from build123d import *

# Parameters (mm, degrees)
SKETCH1_W           = 23
SKETCH1_H           = 31
BOSS_EXTRUDE1_DEPTH = 4
SKETCH2_W           = 10
SKETCH2_H           = 31
BOSS_EXTRUDE2_DEPTH = 2
SKETCH3_R           = 1
CUT_EXTRUDE1_DEPTH  = 24
FILLET1_R           = 2
FILLET2_R           = 6
FILLET3_R           = 0.762


with BuildPart() as part:
    # Sketch1 → Boss-Extrude1 (new body)
    with BuildSketch(Plane.XY):
        Rectangle(SKETCH1_W, SKETCH1_H)
    extrude(amount=BOSS_EXTRUDE1_DEPTH)

    # Sketch2 → Boss-Extrude2 (add)
    with BuildSketch(Plane(origin=(11.5, 0, 0), x_dir=(0, 0, -1), z_dir=(1, 0, 0))):
        with Locations((-9, 0)):
            Rectangle(SKETCH2_W, SKETCH2_H)
    boss_extrude2 = extrude(amount=-BOSS_EXTRUDE2_DEPTH)

    # Mirror1: Boss-Extrude2 across plane
    add(boss_extrude2.mirror(Plane(origin=(0, 0, 0), x_dir=(0, 0, 1), z_dir=(1, 0, 0))))

    # Sketch3 → Cut-Extrude1 (cut, through all)
    with BuildSketch(Plane(origin=(11.5, 0, 0), x_dir=(0, 0, -1), z_dir=(1, 0, 0))):
        with Locations((-12, -8.5)):
            Circle(SKETCH3_R)
        with Locations((-12, -13.5)):
            Circle(SKETCH3_R)
    extrude(amount=-CUT_EXTRUDE1_DEPTH, mode=Mode.SUBTRACT)

    # Fillet1
    fillet1_edges = [part.edges().sort_by_distance(p)[0] for p in [
        (10.5, -15.5, 14),
        (-10.5, -15.5, 14),
    ]]
    fillet(fillet1_edges, radius=FILLET1_R)

    # Fillet2
    fillet2_edges = [part.edges().sort_by_distance(p)[0] for p in [
        (10.5, 15.5, 14),
        (-10.5, 15.5, 14),
    ]]
    fillet(fillet2_edges, radius=FILLET2_R)

    # Fillet3
    fillet3_edges = [part.edges().sort_by_distance(p)[0] for p in [
        (9.5, 0, 4),
        (-9.5, 0, 4),
    ]]
    fillet(fillet3_edges, radius=FILLET3_R)


solid = part.part
Read the model definition and answer for the solid it produces. Units are mm, in the model's axes. A direction names the side the tool comes from. Give positions to 0.01 mm unless a question says otherwise; leave off trailing zeros. Write each loop counter-clockwise with the first axis right and the second up, starting at its lowest first coordinate (ties: lowest second). Pieces come first, ordered by that corner, then holes. Notation, with made-up numbers: (-30, 57.5) -> (14, 57.5) arc R33 ccw to (14, 91.5) -> close; hole circle Ø10 at (-37, 87). An arc over 180 degrees is marked (long way). Answer as a JSON object with one key per item and string values. Group by question number.
1) Find section B-B (y = -8.5). Write down the section's boundary in (x, z).
2) Each of these flat-tipped pins is pushed along its axis until it touches: P1, Ø10, axis at x = -3, y = 0.5, coming from the +Z side; P2, Ø1.5, axis at x = -2, z = 6.5, coming from the -Y side; P3, Ø2.5, axis at y = -8.5, z = 12, coming from the +X side. Where does it stop, or does it pass through?
3) The mould has two halves that part along Y. Classify faces 1 (the cylindrical face through (-10.486, 13.696, 12.289)), 2 (the cylindrical face through (10.51, -7.51, 12.13)), 3 (the flat face through (-11.5, 0, 7)): +Y half, -Y half, draft (parallel to the pull), parting line (faces both ways), or undercut.
4) Find section C-C (y = 2.5). Write down the section's boundary in (x, z).
5) A tool of negligible diameter and unlimited length cuts with its end or side. For faces 4 (the flat face through (0, 15.5, 2)), 5 (the flat face through (9.5, 0, 9)), from which of +Z, -Z, +X, -X, +Y, -Y can it reach the whole face along a straight path? Write none if from no direction.
6) Consider L1, parallel to X at y = 13, z = 9; L2, parallel to Z at x = 1, y = 12; L3, parallel to Y at x = 10.75, z = 12. Determine where each line is inside the solid, lowest interval first. Write a range as from..to.
7) Find section A-A (z = 7). Write down the section's boundary in (x, y).
8) Find section D-D (x = -4). Write down the section's boundary in (y, z), and give its area (3 significant figures).
Values follow:
{
 "1": {"outline": "(-11.5, 0) -> (11.5, 0) -> (11.5, 11) -> (9.5, 11) -> (9.5, 4.76) arc R0.76 cw to (8.74, 4) -> (-8.74, 4) arc R0.76 cw to (-9.5, 4.76) -> (-9.5, 11) -> (-11.5, 11) -> close; (-11.5, 13) -> (-9.5, 13) -> (-9.5, 14) -> (-11.5, 14) -> close; (9.5, 13) -> (11.5, 13) -> (11.5, 14) -> (9.5, 14) -> close"},
 "2": {"P1": "stops at z = 4", "P2": "passes through", "P3": "stops at x = 11.5"},
 "3": {"face 1": "+Y half", "face 2": "undercut", "face 3": "draft"},
 "4": {"outline": "(-11.5, 0) -> (11.5, 0) -> (11.5, 14) -> (9.5, 14) -> (9.5, 4.76) arc R0.76 cw to (8.74, 4) -> (-8.74, 4) arc R0.76 cw to (-9.5, 4.76) -> (-9.5, 14) -> (-11.5, 14) -> close"},
 "5": {"face 4": "+Z, -Z, +X, -X, +Y", "face 5": "+Z, +Y, -Y"},
 "6": {"L1": "x = -11.5..-9.5, 9.5..11.5", "L2": "z = 0..4", "L3": "y = -15.5..-14.5, -12.5..-9.5, -7.5..13.97"},
 "7": {"outline": "(-11.5, -15.5) -> (-9.5, -15.5) -> (-9.5, 15.5) -> (-11.5, 15.5) -> close; (9.5, -15.5) -> (11.5, -15.5) -> (11.5, 15.5) -> (9.5, 15.5) -> close"},
 "8": {"outline": "(-15.5, 0) -> (15.5, 0) -> (15.5, 4) -> (-15.5, 4) -> close", "area": "124 mm2"}
}
